```python
from build123d import *

# Parameters (mm, degrees)
SKETCH1_W           = 630
SKETCH1_H           = 400
EXTRUSION_DEPTH     = 170
DRAWER_S_INTERIOR_T = -12.2428
SKETCH3_W           = 666.2428
SKETCH3_H           = 184
BOSS_EXTRUDE3_DEPTH = 16.5


with BuildPart() as part:
    # Sketch1 → Extrusion (new body)
    with BuildSketch(Plane(origin=(0, 0, 0), x_dir=(1, 0, 0), z_dir=(0, 1, 0))):
        Rectangle(SKETCH1_W, SKETCH1_H)
    extrude(amount=EXTRUSION_DEPTH)

    # Drawer's interior
    drawer_s_interior_openings = [part.faces().sort_by_distance(p)[0] for p in [
        (0, 170, 0),
    ]]
    offset(amount=DRAWER_S_INTERIOR_T, openings=drawer_s_interior_openings, kind=Kind.INTERSECTION)

    # Sketch3 → Boss-Extrude3 (add)
    with BuildSketch(Plane.XY.offset(200)):
        with Locations((5.1214, 92)):
            Rectangle(SKETCH3_W, SKETCH3_H)
    extrude(amount=BOSS_EXTRUDE3_DEPTH)


solid = part.part
```
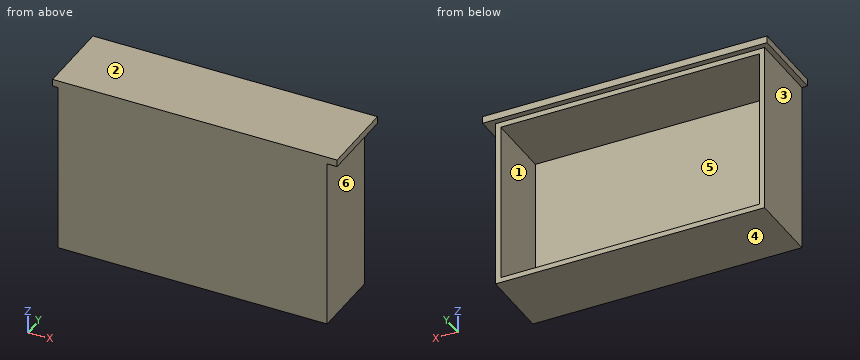
Read the model definition and answer for the solid it produces. Units are mm, in the model's axes. Face numbers are marked on the shaded views. A direction names the side the tool comes from. Coordinates: 2 decimals unless noted, no trailing zeros. Loops run counter-clockwise (first coordinate to the right, second up) from the corner with the lowest first, then second, coordinate; pieces in that order, holes last.
(1) The part is cut by section C-C (z = -156). Determine the outline of the cut face in (x, y), and give its area (3 significant figures).
Solution:
outline: (-315, 0) - (315, 0) - (315, 170) - (302.76, 170) - (302.76, 12.24) - (-302.76, 12.24) - (-302.76, 170) - (-315, 170) - close
area: 11,600 mm2
(2) A tool of negligible diameter and unlimited length cuts with its end or side. For the marked faces 1, 2 and 3, from which of +Z, -Z, +X, -X, +Y, -Y can it reach the whole face along a straight path? Write none if from no direction.
Solution:
face 1: +Y
face 2: +Z, +X, -X, +Y, -Y
face 3: -Z, -X, +Y, -Y
(3) Consider line 1 along X through (y, z) = (138.5, 10.5); line 2 along Z through (x, y) = (-131, 90.5); line 3 along Y through (x, z) = (94.5, -36). Determine where each line is inside the solid, lowest interval first.
Solution:
line 1: x = -315 to -302.76, 302.76 to 315
line 2: z = -200 to -187.76, 187.76 to 216.5
line 3: y = 0 to 12.24
(4) Flat-ended cylindrical pins translate along their axes: pin 1 Ø3 at (y, z) = (149, -124) entering from -X; pin 2 Ø10 at (x, z) = (97.5, -97.5) entering from -Y; pin 3 Ø2 at (x, z) = (-10.5, -78) entering from +Y; pin 4 Ø6 at (y, z) = (152, 59.5) entering from +X. Find the tip coordinate at first contact, or state that the pin passes through.
Solution:
pin 1: stops at x = -315
pin 2: stops at y = 0
pin 3: stops at y = 12.24
pin 4: stops at x = 315
(5) The mould has two halves that part along Z. Classify the marked faces 4, 5 and 6: released by +Z, released by -Z, zero draft, split by the parting line, or undercut.
Solution:
face 4: released by -Z
face 5: undercut
face 6: zero draft
(6) The part is cut by section A-A (x = 285). Determine the outline of the cut face in (y, z).
Solution:
outline: (0, -200) - (170, -200) - (170, -187.76) - (12.24, -187.76) - (12.24, 187.76) - (170, 187.76) - (170, 200) - (184, 200) - (184, 216.5) - (0, 216.5) - close
(7) The part is cut by section B-B (y = 41.5). Determine the outline of the cut face in (x, z), and give its area (3 significant figures).
Solution:
outline: (-328, 200) - (-315, 200) - (-315, -200) - (315, -200) - (315, 200) - (338.24, 200) - (338.24, 216.5) - (-328, 216.5) - close; hole (-302.76, -187.76) - (302.76, -187.76) - (302.76, 187.76) - (-302.76, 187.76) - close
area: 35,600 mm2
